For this review, take the finished solid that the model builds, in its own axes (mm). Face numbers are marked on the shaded views. Coordinates: 2 decimals unless noted, no trailing zeros. Write each loop counter-clockwise with the first axis right and the second up, starting at its lowest first coordinate (ties: lowest second). Pieces come first, ordered by that corner, then holes.
```python
from build123d import *

# Parameters (mm, degrees)
EXTRUDE_4_DEPTH     = 15
SKETCH_3_R          = 10
CUT_EXTRUDE_1_DEPTH = 2


with BuildPart() as part:
    # ｽｹｯﾁ2 → ﾎﾞｽ - 押し出し4 (new body)
    with BuildSketch(Plane(origin=(0, 0, 0), x_dir=(1, 0, 0), z_dir=(0, 1, 0))):
        with BuildLine():
            ThreePointArc((-53.82643789, -36.437818048), (-56.846261527, -34.367935813), (-60.466933112, -34.910600109))
            Line((-60.466933112, -34.910600109), (-64.807406984, -37.416573868))
            ThreePointArc((-64.807406984, -37.416573868), (-67.177509772, -40.614402853), (-66.461234116, -44.529814279))
            ThreePointArc((-66.461234116, -44.529814279), (49.665387485, -62.716419588), (58.57572973, 54.487465409))
            Line((58.57572973, 54.487465409), (57.289371136, 55.838409315))
            Line((57.289371136, 55.838409315), (25.911523347, 88.791671712))
            ThreePointArc((25.911523347, 88.791671712), (19.306695871, 93.382511176), (11.427401304, 95))
            Line((11.427401304, 95), (0, 95))
            ThreePointArc((0, 95), (-15, 80), (0, 65))
            ThreePointArc((0, 65), (57.41714976, -30.467538684), (-53.82643789, -36.437818048))
        make_face()
    extrude(amount=EXTRUDE_4_DEPTH)

    # ｽｹｯﾁ3 → ｶｯﾄ - 押し出し1 (cut)
    with BuildSketch(Plane(origin=(0, 15, 0), x_dir=(1, 0, 0), z_dir=(0, 1, 0))):
        with Locations(Location((0, 80, 0), (0, 0, 270))):
            Circle(SKETCH_3_R)
    extrude(amount=-CUT_EXTRUDE_1_DEPTH, mode=Mode.SUBTRACT)


solid = part.part
```
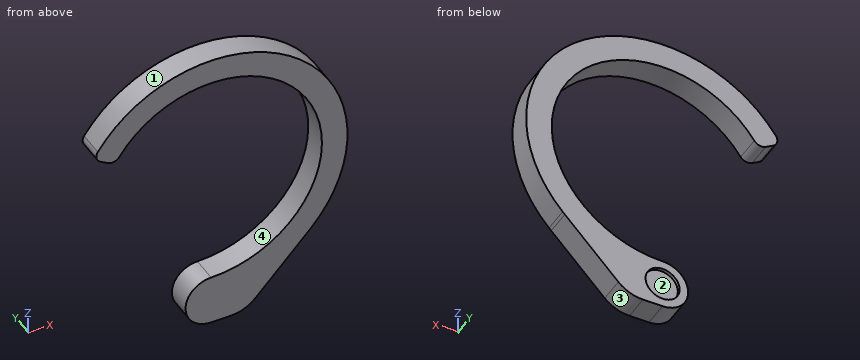
1) For L1, parallel to X at y = 13.75, z = -80; L2, parallel to Z at x = 0, y = 7.5; L3, parallel to Z at x = -10.5, y = 5.5, list the stretches that pass through material, from the lowest coordinate up.
2) The part is to be moulded in two halves that separate along Z. For the marked faces 1, 2, 3 and 4, say which applies: pulls with the +Z half, pulls with the -Z half, needs draft (parallel to the pull), parting line crosses it, or undercut.
3) Consider section D-D (x = -40). Give the boundary of the cut face in (y, z), then the cut area to 3 significant figures.
4) Consider section C-C (z = 0). Give the boundary of the cut face in (x, y).
5) Clearance check with flat-ended pins moving along their axes: P1, Ø6, axis at x = -3, z = -77.5, coming from the +Y side; P2, Ø8, axis at x = 52, y = 6.5, coming from the +Z side; P3, Ø5, axis at y = 3.5, z = 33.5, coming from the -X side. State where each tip first meets the part, or that it passes through.
6) Consider section B-B (x = 37). Give the boundary of the cut face in (y, z), then the cut area to 3 significant figures.
7) Consider section A-A (y = 6.25). Give the boundary of the cut face in (x, z).
Results:
1. L1: x = -15 to -10, 10 to 34.28
1. L2: z = -95 to -65, 65 to 80
1. L3: z = -90.71 to -69.29, 64.15 to 79.31
2. face 1: parting line crosses it
2. face 2: undercut
2. face 3: pulls with the -Z half
2. face 4: undercut
3. outline: (0, 51.23) - (15, 51.23) - (15, 69.28) - (0, 69.28) - close
3. area: 271 mm2
4. outline: (65, 0) - (80, 0) - (80, 15) - (65, 15) - close
5. P1: stops at y = 13
5. P2: stops at z = 64
5. P3: stops at x = -62.35
6. outline: (0, -77.15) - (15, -77.15) - (15, -53.44) - (0, -53.44) - close; (0, 53.44) - (15, 53.44) - (15, 70.93) - (0, 70.93) - close
6. area: 618 mm2
7. outline: (-66.46, 44.53) arc R5 ccw to (-64.81, 37.42) - (-60.47, 34.91) arc R5 ccw to (-53.83, 36.44) arc R65 cw (long way) to (0, -65) arc R15 ccw to (0, -95) - (11.43, -95) arc R20 ccw to (25.91, -88.79) - (58.58, -54.49) arc R80 ccw (long way) to start
